Build history of the part. All positions in model axes, mm. Give positions to 0.01 mm unless a question says otherwise; leave off trailing zeros. Loops run counter-clockwise (first coordinate to the right, second up) from the corner with the lowest first, then second, coordinate; pieces in that order, holes last. Notation, with made-up numbers: (49, -19.5) -> (63, -19.5) arc R26 ccw to (63, 9.5) -> close; hole circle Ø2 at (24.5, -3). An arc over 180 degrees is marked (long way). Answer as a JSON object with one key per item and string values. Group by question number.
Q1. Band-saw the part on B-B, the plane z = 88. Write the cut outline in (x, y), plus the area to 3 significant figures.
Q2. Band-saw the part on C-C, the plane x = -70. Write the cut outline in (y, z).
Q3. Band-saw the part on A-A, the plane y = 0.8. Write the cut outline in (x, z), plus the area to 3 significant figures.
Q4. Wall check: probe 1 along Z at (x, y) = (-41, 0.4); probe 2 along X at (y, z) = (0.75, -67); probe 3 along X at (y, z) = (0.6, 47). Give the ranges that are in metal, low to high. Write a range as from..to.
Q5. Drop a flat-ended pin along its axis: pin 1 (4.5 mm diameter, centred on x = -79, z = 39.47, fed in from -Y). Give the stop position or say it passes through.
Q6. Two-plate mould, pull along X, no slides. Class faces 1 (the cylindrical face through (76.84, 0.51, -47.27)), 2 (the cylindrical face through (44.87, 0.49, -104.21)), 3 (the flat face through (-1, 0, -1)): pulls with the +X half, pulls with the -X half, needs draft (parallel to the pull), parting line crosses it, or undercut.
from build123d import *

# Parameters (mm, degrees)
BOSS_EXTRUDE1_DEPTH = 1
SKETCH2_R           = 2.5
CUT_EXTRUDE1_DEPTH  = 1


with BuildPart() as part:
    # Sketch1 → Boss-Extrude1 (new body)
    with BuildSketch(Plane(origin=(0, 0, 0), x_dir=(1, 0, 0), z_dir=(0, 1, 0))):
        with BuildLine():
            Line((83, -33.574175964), (83, 42.632037736))
            ThreePointArc((83, 42.632037736), (82.612487462, 45.388862866), (81.47998304, 47.932027136))
            Line((81.47998304, 47.932027136), (48.437506625, 100.7999894))
            ThreePointArc((48.437506625, 100.7999894), (44.805208909, 104.246424812), (39.957523585, 105.5))
            Line((39.957523585, 105.5), (-39.957523585, 105.5))
            ThreePointArc((-39.957523585, 105.5), (-44.805208909, 104.246424812), (-48.437506625, 100.7999894))
            Line((-48.437506625, 100.7999894), (-81.47998304, 47.932027136))
            ThreePointArc((-81.47998304, 47.932027136), (-82.612487462, 45.388862866), (-83, 42.632037736))
            Line((-83, 42.632037736), (-83, -33.574175964))
            ThreePointArc((-83, -33.574175964), (-82.819563867, -35.465251176), (-82.284766909, -37.288082728))
            Line((-82.284766909, -37.288082728), (-57.514437295, -99.213906764))
            ThreePointArc((-57.514437295, -99.213906764), (-53.835958479, -103.780672305), (-48.229670386, -105.5))
            Line((-48.229670386, -105.5), (48.229670386, -105.5))
            ThreePointArc((48.229670386, -105.5), (53.835958479, -103.780672305), (57.514437295, -99.213906764))
            Line((57.514437295, -99.213906764), (82.284766909, -37.288082728))
            ThreePointArc((82.284766909, -37.288082728), (82.819563867, -35.465251176), (83, -33.574175964))
        make_face()
    extrude(amount=BOSS_EXTRUDE1_DEPTH)

    # Sketch2 → Cut-Extrude1 (cut)
    with BuildSketch(Plane(origin=(0, 1, 0), x_dir=(1, 0, 0), z_dir=(0, 1, 0))):
        with Locations((79, 48.528930886)):
            Circle(SKETCH2_R)
        with Locations((79, -39.471069114)):
            Circle(SKETCH2_R)
        with Locations((-79, 48.528930886)):
            Circle(SKETCH2_R)
        with Locations((-79, -39.471069114)):
            Circle(SKETCH2_R)
    extrude(amount=-CUT_EXTRUDE1_DEPTH, mode=Mode.SUBTRACT)


solid = part.part
Worked answers:
{
 "1": {"outline": "(-62, 0) -> (62, 0) -> (62, 1) -> (-62, 1) -> close", "area": "124 mm2"},
 "2": {"outline": "(0, -66.3) -> (1, -66.3) -> (1, 68) -> (0, 68) -> close"},
 "3": {"outline": "(-83, -42.63) arc R10 ccw to (-81.48, -47.93) -> (-81.44, -47.99) arc R2.5 cw (long way) to (-79.59, -50.96) -> (-48.44, -100.8) arc R10 ccw to (-39.96, -105.5) -> (39.96, -105.5) arc R10 ccw to (48.44, -100.8) -> (79.59, -50.96) arc R2.5 cw (long way) to (81.44, -47.99) -> (81.48, -47.93) arc R10 ccw to (83, -42.63) -> (83, 33.57) arc R10 ccw to (82.28, 37.29) -> (81.49, 39.27) arc R2.5 cw (long way) to (80.67, 41.34) -> (57.51, 99.21) arc R10 ccw to (48.23, 105.5) -> (-48.23, 105.5) arc R10 ccw to (-57.51, 99.21) -> (-80.67, 41.34) arc R2.5 cw (long way) to (-81.49, 39.27) -> (-82.28, 37.29) arc R10 ccw to (-83, 33.57) -> close", "area": "30,700 mm2"},
 "4": {"probe 1": "-105.45..105.5", "probe 2": "-69.56..69.56", "probe 3": "-78.4..78.4"},
 "5": {"pin 1": "through"},
 "6": {"face 1": "undercut", "face 2": "pulls with the +X half", "face 3": "needs draft"}
}
